Job drawing, mm, ordinate dimensions from the low corner. One solid piece. A direction names the side the tool comes from. Give positions to 0.01 mm unless a question says otherwise; leave off trailing zeros. Loops run counter-clockwise (first coordinate to the right, second up) from the corner with the lowest first, then second, coordinate; pieces in that order, holes last. Notation, with made-up numbers: M 0.25,1 L 53.25,1 A14 ccw 53.25,11 Z; hole C 48,21 d11. An arc over 180 degrees is marked long. Answer in a Markdown table with one row per item.
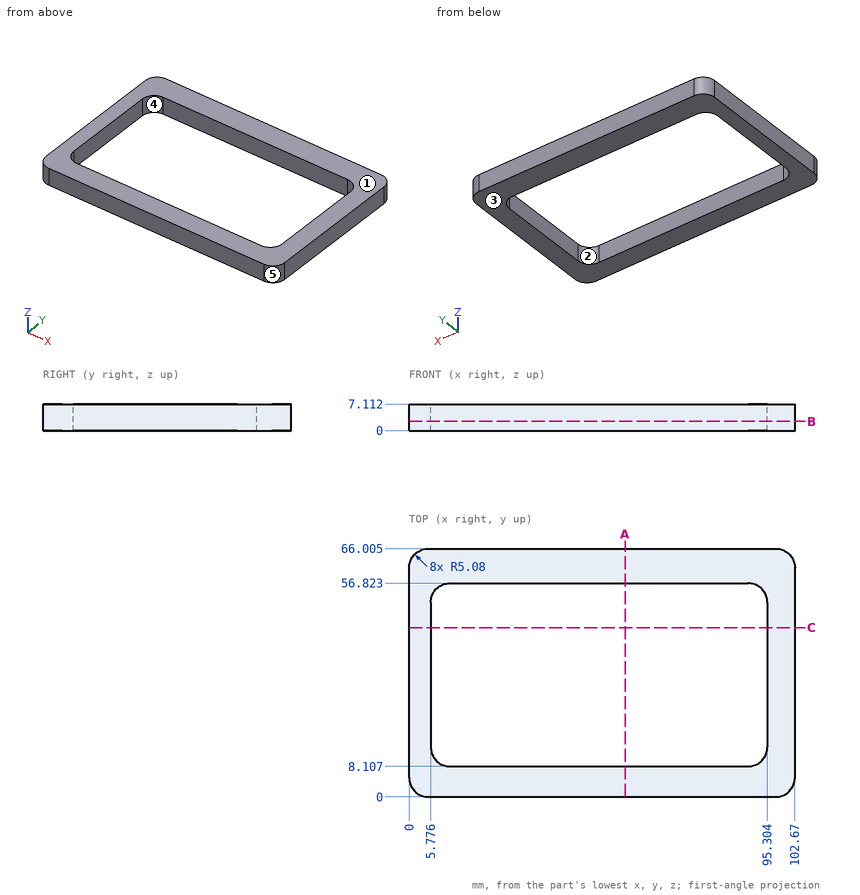
(1) Saw through at C-C (y = 45). Write the cut outline in (x, z).
Recorded:
| item | result |
|---|---|
| outline | M 0,0 L 5.78,0 L 5.78,7.11 L 0,7.11 Z; M 95.3,0 L 102.67,0 L 102.67,7.11 L 95.3,7.11 Z |
(2) Saw through at B-B (z = 2.5). Write the cut outline in (x, y) (1 decimal).
Recorded:
| item | result |
|---|---|
| outline | M 0,5.1 A5.1 ccw 5.1,0 L 97.6,0 A5.1 ccw 102.7,5.1 L 102.7,60.9 A5.1 ccw 97.6,66 L 5.1,66 A5.1 ccw 0,60.9 Z; hole M 5.8,13.2 A5.1 ccw 10.9,8.1 L 90.2,8.1 A5.1 ccw 95.3,13.2 L 95.3,51.7 A5.1 ccw 90.2,56.8 L 10.9,56.8 A5.1 ccw 5.8,51.7 Z |
(3) Pin check, flat tips, straight feed: pin 1 Ø4 at (x, z) = (12, 4.5) entering from -Y; pin 2 Ø12 at (x, y) = (73, 16) entering from +Z. Stop position of each tip, or through.
Recorded:
| item | result |
|---|---|
| pin 1 | stops at y = 0 |
| pin 2 | passes through |
(4) Drill centre lines: line 1 along X through (y, z) = (24, 6); line 2 along Y through (x, z) = (69, 4.25) (1 decimal); line 3 along X through (y, z) = (61, 1.75). Where is each one in solid material? Low to high.
Recorded:
| item | result |
|---|---|
| line 1 | x = 0 to 5.78, 95.3 to 102.67 |
| line 2 | y = 0 to 8.1, 56.8 to 66 |
| line 3 | x = 0 to 102.67 |
(5) Pull direction Y, two halves, no side cores. Call the marked faces 3, 4 and 5: +Y half, -Y half, draft (parallel to the pull), parting line (faces both ways), or undercut.
Recorded:
| item | result |
|---|---|
| face 3 | draft |
| face 4 | undercut |
| face 5 | -Y half |
(6) Which spindle directions (+Z, -Z, +X, -X, +Y, -Y) get a long thin tool onto all of the face, cutting with end or side? Do the marked faces 1 and 2. Say none if no direction does.
Recorded:
| item | result |
|---|---|
| face 1 | +Z, +X, -X, +Y, -Y |
| face 2 | +Z, -Z |
(7) Saw through at A-A (x = 57.5). Write the cut outline in (y, z) (1 decimal).
Recorded:
| item | result |
|---|---|
| outline | M 0,0 L 8.1,0 L 8.1,7.1 L 0,7.1 Z; M 56.8,0 L 66,0 L 66,7.1 L 56.8,7.1 Z |
